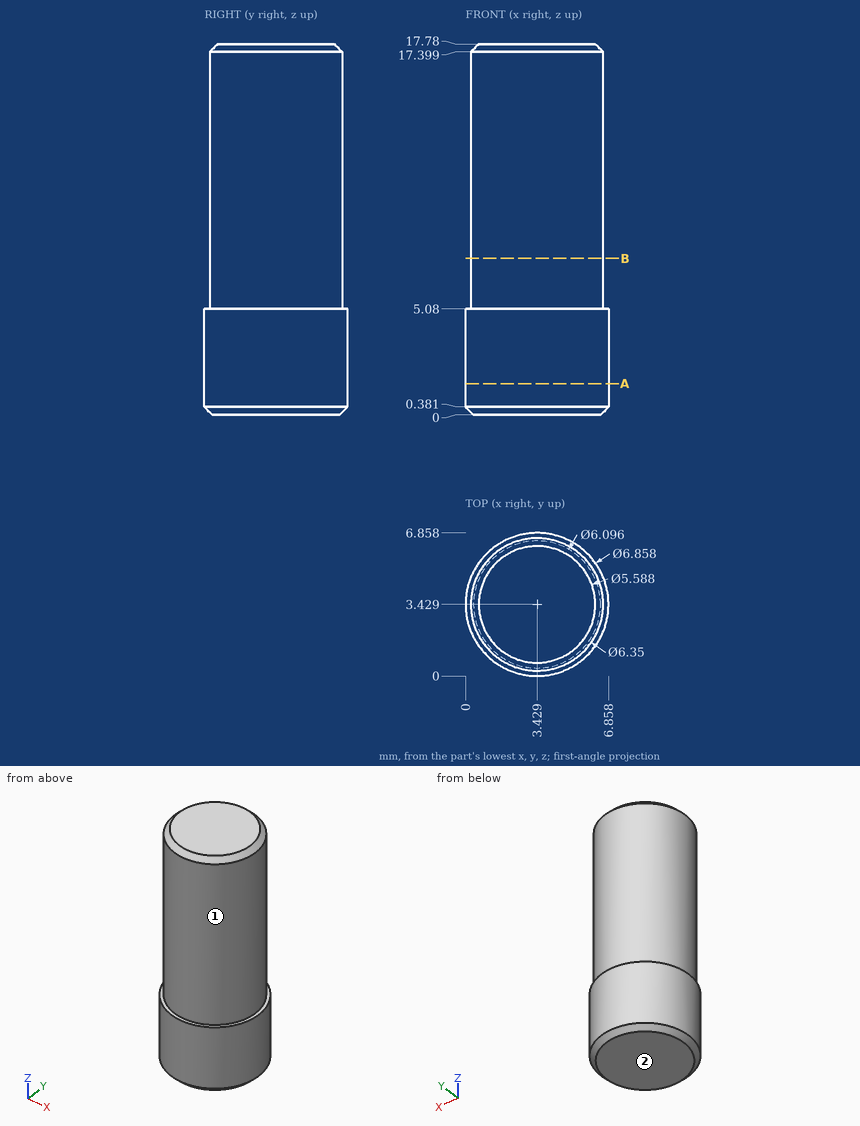
Can you work these out from the drawing? Everything is in mm from the part's minimum corner. Give positions to 0.01 mm unless a question says otherwise; leave off trailing zeros. Write each loop counter-clockwise with the first axis right and the second up, starting at its lowest first coordinate (ties: lowest second). Pieces come first, ordered by that corner, then holes. Notation, with made-up numbers: (-14, 27) -> (-2, 27) arc R13 cw to (-2, 34) -> close; hole circle Ø9 at (-2.75, 76). An arc over 180 degrees is marked (long way). Write each question's results on one line, items separated by ' | '. Start each with the question number.
Q1. We'd pull the mould along Y, two halves only. Please class the marked faces 1 and 2: +Y half, -Y half, draft (parallel to the pull), parting line (faces both ways), or undercut.
Q2. Suppose I cut it at A-A, the plane z = 1.5. List the corners of the cut face in (x, y) for me, and give its area (3 significant figures).
Q3. I'm going to push flat-ended pins straight in: pin 1 Ø1 at (y, z) = (2, 7.5) entering from -X; pin 2 Ø3 at (x, z) = (5, 11) entering from +Y; pin 3 Ø1.5 at (x, z) = (6, 4) entering from +Y. Where does each tip first touch, or does it pass through?
Q4. I need wall thicknesses on probe 1 along X at (y, z) = (3.25, 3); probe 2 along Y at (x, z) = (6.25, 15.5); probe 3 along X at (y, z) = (5.75, 2.25). Which ranges of each line are inside material? Lowest first, please.
Q5. Suppose I cut it at B-B, the plane z = 7.5. List the corners of the cut face in (x, y) for me (3 decimals).
Outcome:
1) face 1: parting line | face 2: draft
2) outline: circle Ø6.86 at (3.43, 3.43) | area: 36.9 mm2
3) pin 1: x = 0.39 | pin 2: y = 6.6 | pin 3: y = 6.33
4) probe 1: 0 to 6.85 | probe 2: 1.97 to 4.89 | probe 3: 0.9 to 5.95
5) outline: circle Ø6.35 at (3.429, 3.429)
